Here's the drawing with two shaded views (mm, measured from the low corner). I have some questions. Round coordinates to 2 decimals unless told otherwise and drop trailing zeros. Loops run counter-clockwise (first coordinate to the right, second up) from the corner with the lowest first, then second, coordinate; pieces in that order, holes last.
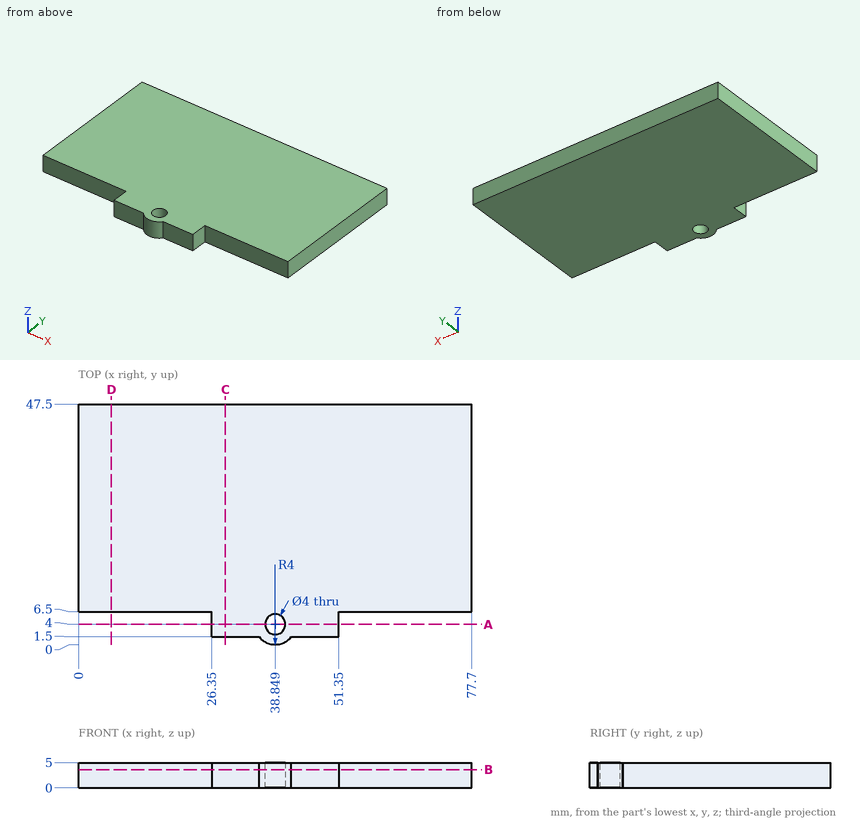
Item 1: Will this pin go through, and if not, where does the flat tip stop? pin 1 (2.5 mm diameter, centred on x = 64.5, z = 2.5, fed in from -Y).
Results list:
pin 1: stops at y = 6.5
Item 2: If we section it at D-D, the plane x = 6.5: Please give me the cut outline in (y, z), then the cut area to 3 significant figures.
Results list:
outline: (6.5, 0) - (47.5, 0) - (47.5, 5) - (6.5, 5) - close
area: 205 mm2
Item 3: If I drill on line 1 along Y through (x, z) = (17.5, 2.8); line 2 along Y through (x, z) = (47, 1.3); line 3 along Y through (x, z) = (38.5, 4.05) (1 decimal), over which ranges is the centre line in solid material (lowest first)?
Results list:
line 1: y = 6.5 to 47.5
line 2: y = 1.5 to 47.5
line 3: y = 0 to 2, 6 to 47.5
Item 4: If we section it at B-B, the plane z = 3.6: Please give me the cut outline in (x, y).
Results list:
outline: (0, 6.5) - (26.35, 6.5) - (26.35, 1.5) - (35.73, 1.5) arc R4 ccw to (41.97, 1.5) - (51.35, 1.5) - (51.35, 6.5) - (77.7, 6.5) - (77.7, 47.5) - (0, 47.5) - close; hole circle Ø4 at (38.85, 4)
Item 5: If we section it at C-C, the plane x = 29: Please give me the cut outline in (y, z), then the cut area to 3 significant figures.
Results list:
outline: (1.5, 0) - (47.5, 0) - (47.5, 5) - (1.5, 5) - close
area: 230 mm2
Item 6: If we section it at A-A, the plane y = 4: Please give me the cut outline in (x, z).
Results list:
outline: (26.35, 0) - (36.85, 0) - (36.85, 5) - (26.35, 5) - close; (40.85, 0) - (51.35, 0) - (51.35, 5) - (40.85, 5) - close
